Work out the finished part from the listing and answer in its coordinate system (mm). A direction names the side the tool comes from. Coordinates: 2 decimals unless noted, no trailing zeros. Loops run counter-clockwise (first coordinate to the right, second up) from the corner with the lowest first, then second, coordinate; pieces in that order, holes last. Notation, with made-up numbers: (48.25, -2) -> (82.25, -2) arc R23 ccw to (82.25, 23) -> close; hole circle Ø8 at (7, -9.75). An arc over 180 degrees is marked (long way). Use a Markdown table: item, result.
from build123d import *

# Parameters (mm, degrees)
SKETCH1_W           = 24.94
SKETCH1_H           = 6
BOSS_EXTRUDE1_DEPTH = 3
SKETCH2_W           = 4.65
SKETCH2_H           = 6
BOSS_EXTRUDE2_DEPTH = 7
SKETCH3_R           = 1.615
CUT_EXTRUDE1_DEPTH  = 4
CHAMFER2_SIZE       = 2.2


with BuildPart() as part:
    # Sketch1 → Boss-Extrude1 (new body)
    with BuildSketch(Plane(origin=(0, 0, 0), x_dir=(1, 0, 0), z_dir=(0, 1, 0))):
        Rectangle(SKETCH1_W, SKETCH1_H)
    extrude(amount=BOSS_EXTRUDE1_DEPTH)

    # Sketch2 → Boss-Extrude2 (add)
    with BuildSketch(Plane(origin=(0, 3, 0), x_dir=(1, 0, 0), z_dir=(0, 1, 0))):
        with Locations((-3.715, 0)):
            Rectangle(SKETCH2_W, SKETCH2_H)
    boss_extrude2 = extrude(amount=BOSS_EXTRUDE2_DEPTH)

    # Sketch3 → Cut-Extrude1 (cut, through all)
    with BuildSketch(Plane(origin=(0, 3, 0), x_dir=(1, 0, 0), z_dir=(0, 1, 0))):
        with Locations((-9.335, 0)):
            Circle(SKETCH3_R)
    cut_extrude1 = extrude(amount=-CUT_EXTRUDE1_DEPTH, mode=Mode.SUBTRACT)

    # Mirror1: Boss-Extrude2, Cut-Extrude1 across plane
    add(boss_extrude2.mirror(Plane(origin=(0, 0, 0), x_dir=(0, 0, 1), z_dir=(1, 0, 0))))
    add(cut_extrude1.mirror(Plane(origin=(0, 0, 0), x_dir=(0, 0, 1), z_dir=(1, 0, 0))), mode=Mode.SUBTRACT)

    # Chamfer2
    chamfer2_edges = [part.edges().sort_by_distance(p)[0] for p in [
        (12.47, 1.5, 3),
        (12.47, 1.5, -3),
    ]]
    chamfer(chamfer2_edges, length=CHAMFER2_SIZE)


solid = part.part
Q1. Section C-C on y = 2 is taken. Determine the outline of the cut face in (x, z) (3 decimals).
Solved:
| item | result |
|---|---|
| outline | (-12.47, -3) -> (10.27, -3) -> (12.47, -0.8) -> (12.47, 0.8) -> (10.27, 3) -> (-12.47, 3) -> close; hole circle Ø3.23 at (-9.335, 0); hole circle Ø3.23 at (9.335, 0) |
Q2. Consider line 1 (X direction, y = 1.75, z = 0); line 2 (X direction, y = 6.5, z = -0.5); line 3 (X direction, y = 1.75, z = 0.75). Determine where each line is inside the solid, lowest interval first. Write a range as [from, to].
Solved:
| item | result |
|---|---|
| line 1 | [-12.47, -10.95], [-7.72, 7.72], [10.95, 12.47] |
| line 2 | [-6.04, -1.39], [1.39, 6.04] |
| line 3 | [-12.47, -10.77], [-7.9, 7.9], [10.77, 12.47] |
Q3. Section A-A on z = 0 is taken. Determine the outline of the cut face in (x, y), and give its area (3 significant figures).
Solved:
| item | result |
|---|---|
| outline | (-12.47, 0) -> (-10.95, 0) -> (-10.95, 3) -> (-12.47, 3) -> close; (-7.72, 0) -> (7.72, 0) -> (7.72, 3) -> (6.04, 3) -> (6.04, 10) -> (1.39, 10) -> (1.39, 3) -> (-1.39, 3) -> (-1.39, 10) -> (-6.04, 10) -> (-6.04, 3) -> (-7.72, 3) -> close; (10.95, 0) -> (12.47, 0) -> (12.47, 3) -> (10.95, 3) -> close |
| area | 121 mm² |
Q4. Section B-B on y = 8.5 is taken. Determine the outline of the cut face in (x, z), and give its area (3 significant figures).
Solved:
| item | result |
|---|---|
| outline | (-6.04, -3) -> (-1.39, -3) -> (-1.39, 3) -> (-6.04, 3) -> close; (1.39, -3) -> (6.04, -3) -> (6.04, 3) -> (1.39, 3) -> close |
| area | 55.8 mm² |
Q5. For faces 1 (the flat face through (-1.39, 6, 0)), 2 (the flat face through (7.8, 3, 1.3)), 3 (the flat face through (-6.04, 6, 0)), determine the directions among +Z, -Z, +X, -X, +Y, -Y from which every point of the face is accessible in a straight line to the end or side of a thin tool.
Solved:
| item | result |
|---|---|
| face 1 | +Z, -Z, +Y |
| face 2 | +Z, -Z, +X, +Y |
| face 3 | +Z, -Z, -X, +Y |
Q6. Section D-D on z = -2.25 is taken. Determine the outline of the cut face in (x, y).
Solved:
| item | result |
|---|---|
| outline | (-12.47, 0) -> (11.02, 0) -> (11.02, 3) -> (6.04, 3) -> (6.04, 10) -> (1.39, 10) -> (1.39, 3) -> (-1.39, 3) -> (-1.39, 10) -> (-6.04, 10) -> (-6.04, 3) -> (-12.47, 3) -> close |
Q7. Determine the mould class of faces 4 (the flat face through (11.39, 1.48, 1.88)), 5 (the cylindrical face through (-10.95, 1.52, -0.07)), 6 (the flat face through (-4, 10, 0)) for opening direction Z: pulls with the +Z half, pulls with the -Z half, needs draft (parallel to the pull), parting line crosses it, or undercut.
Solved:
| item | result |
|---|---|
| face 4 | pulls with the +Z half |
| face 5 | undercut |
| face 6 | needs draft |
Q8. Given pin 1 Ø3.5 at (x, z) = (-9.335, 0) entering from +Y, flat-ended and moving along its own axis, determine where the tip first touches the part or whether it passes through.
Solved:
| item | result |
|---|---|
| pin 1 | y = 3 |
